Input: dimensioned drawing with shaded views. Units: mm. Origin: part minimum x, y, z. A direction names the side the tool comes from. Give positions to 0.01 mm unless a question says otherwise; leave off trailing zeros. Write each loop counter-clockwise with the first axis right and the second up, starting at its lowest first coordinate (ties: lowest second). Pieces come first, ordered by that corner, then holes.
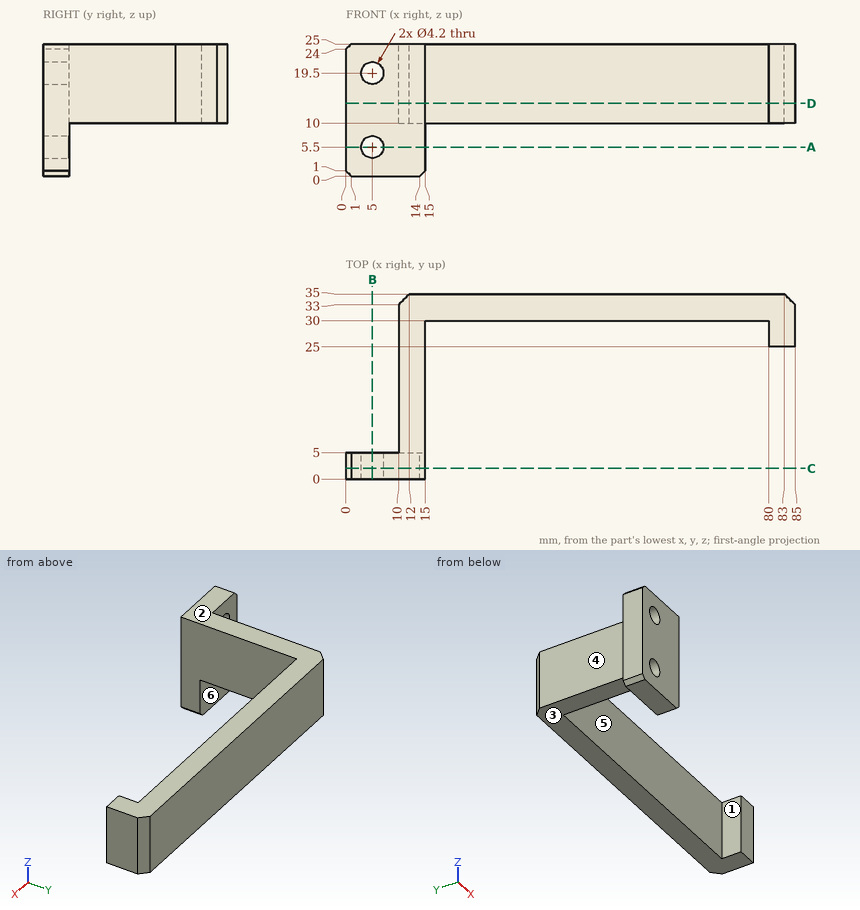
Item 1: Section D-D, the plane z = 13.75. Return the cut outline in (x, y), plus the area to 3 significant figures.
Found:
outline: (0, 0) - (15, 0) - (15, 30) - (80, 30) - (80, 25) - (85, 25) - (85, 33) - (83, 35) - (12, 35) - (10, 33) - (10, 5) - (0, 5) - close
area: 596 mm2
Item 2: Section A-A, the plane z = 5.5. Return the cut outline in (x, y), plus the area to 3 significant figures.
Found:
outline: (0, 0) - (2.9, 0) - (2.9, 5) - (0, 5) - close; (7.1, 0) - (15, 0) - (15, 5) - (7.1, 5) - close
area: 54.0 mm2
Item 3: Reachability of the marked faces 1, 2 and 3 from +Z, -Z, +X, -X, +Y, -Y: full face, straight path, thin tool, end or side. Return the list, or none.
Found:
face 1: +Z, -Z, -Y
face 2: +Z, +X, -X, +Y, -Y
face 3: -Z, +X, -X, +Y
Item 4: Line query: L1, parallel to Z at x = 5, y = 1.3; L2, parallel to X at y = 2.3, z = 19.5; L3, parallel to X at y = 26.5, z = 19.5. Output: solid intervals per line, ascending.
Found:
L1: z = 0 to 3.4, 7.6 to 17.4, 21.6 to 25
L2: x = 0 to 2.9, 7.1 to 15
L3: x = 10 to 15, 80 to 85
Item 5: Section B-B, the plane x = 5. Return the cut outline in (y, z), plus the area to 3 significant figures.
Found:
outline: (0, 0) - (5, 0) - (5, 3.4) - (0, 3.4) - close; (0, 7.6) - (5, 7.6) - (5, 17.4) - (0, 17.4) - close; (0, 21.6) - (5, 21.6) - (5, 25) - (0, 25) - close
area: 83.0 mm2
Item 6: Section C-C, the plane y = 2. Return the cut outline in (x, z).
Found:
outline: (0, 1) - (1, 0) - (14, 0) - (15, 1) - (15, 25) - (1, 25) - (0, 24) - close; hole circle Ø4.2 at (5, 5.5); hole circle Ø4.2 at (5, 19.5)
Item 7: Pull-direction query (X, two-part tool) for the marked faces 4, 5 and 6; classes: +X half, -X half, draft (parallel to the pull), parting line (faces both ways), or undercut.
Found:
face 4: -X half
face 5: undercut
face 6: draft
Item 8: Pin query (flat end, axial travel): pin 1 Ø8 at (x, z) = (29.5, 13) entering from -Y; pin 2 Ø5 at (x, z) = (16, 6.5) entering from +Y; pin 3 Ø3.5 at (x, z) = (5, 5.5) entering from +Y; pin 4 Ø4.5 at (y, z) = (16, 17) entering from -X. Return the tip coordinate at first contact, or that it passes through.
Found:
pin 1: stops at y = 30
pin 2: stops at y = 5
pin 3: passes through
pin 4: stops at x = 10
